```python
from build123d import *

# Parameters (mm, degrees)
SKETCH_1_R      = 1.65
EXTRUDE_1_DEPTH = 4.5


with BuildPart() as part:
    # 草图1 → 凸台-拉伸1 (new body)
    with BuildSketch(Plane.XY):
        with BuildLine():
            Line((7985.952332202, 5156.773837904), (7985.952332202, 5150.976359203))
            ThreePointArc((7985.952332202, 5150.976359203), (7986.043696587, 5150.147298626), (7986.313404682, 5149.358029069))
            Line((7986.313404682, 5149.358029069), (7993.434341187, 5134.194369164))
            ThreePointArc((7993.434341187, 5134.194369164), (8000.767739464, 5133.728654178), (7997.228995286, 5140.168600636))
            Line((7997.228995286, 5140.168600636), (7997.228995286, 5144.169137786))
            ThreePointArc((7997.228995286, 5144.169137786), (7998.107674943, 5146.290458129), (8000.228995286, 5147.169137786))
            Line((8000.228995286, 5147.169137786), (8057.335847124, 5147.169137786))
            ThreePointArc((8057.335847124, 5147.169137786), (8059.457167467, 5146.290458129), (8060.335847124, 5144.169137786))
            Line((8060.335847124, 5144.169137786), (8060.335847124, 5140.181434516))
            ThreePointArc((8060.335847124, 5140.181434516), (8056.672629109, 5133.729954227), (8064.072159737, 5134.266340868))
            Line((8064.072159737, 5134.266340868), (8071.275990148, 5149.357818804))
            ThreePointArc((8071.275990148, 5149.357818804), (8071.552278457, 5150.153987911), (8071.645915883, 5150.991515528))
            Line((8071.645915883, 5150.991515528), (8071.645915883, 5156.773837904))
            ThreePointArc((8071.645915883, 5156.773837904), (8070.767236227, 5158.895158248), (8068.645915883, 5159.773837904))
            Line((8068.645915883, 5159.773837904), (7988.952332202, 5159.773837904))
            ThreePointArc((7988.952332202, 5159.773837904), (7986.831011858, 5158.895158248), (7985.952332202, 5156.773837904))
        make_face()
        with Locations((7997.228995286, 5135.976359203)):
            Circle(SKETCH_1_R, mode=Mode.SUBTRACT)
        with Locations((8005.228995286, 5150.976359203)):
            Circle(SKETCH_1_R, mode=Mode.SUBTRACT)
        with Locations((8052.228995286, 5150.976359203)):
            Circle(SKETCH_1_R, mode=Mode.SUBTRACT)
        with Locations((8013.728995286, 5150.976359203)):
            Circle(SKETCH_1_R, mode=Mode.SUBTRACT)
        with Locations((8043.728995286, 5150.976359203)):
            Circle(SKETCH_1_R, mode=Mode.SUBTRACT)
        with Locations((8060.228995286, 5135.976359203)):
            Circle(SKETCH_1_R, mode=Mode.SUBTRACT)
        with Locations((7989.759553619, 5150.976359203)):
            Circle(SKETCH_1_R, mode=Mode.SUBTRACT)
        with Locations((8067.903645142, 5150.680599992)):
            Circle(SKETCH_1_R, mode=Mode.SUBTRACT)
        with Locations((8025.728995286, 5150.976359203)):
            Circle(SKETCH_1_R, mode=Mode.SUBTRACT)
        with Locations((8031.728995286, 5150.976359203)):
            Circle(SKETCH_1_R, mode=Mode.SUBTRACT)
        with Locations((8005.228995286, 5156.218532456)):
            Circle(SKETCH_1_R, mode=Mode.SUBTRACT)
        with Locations((8052.228995286, 5156.218532456)):
            Circle(SKETCH_1_R, mode=Mode.SUBTRACT)
        with Locations((8013.728995286, 5156.218532456)):
            Circle(SKETCH_1_R, mode=Mode.SUBTRACT)
        with Locations((8043.728995286, 5156.218532456)):
            Circle(SKETCH_1_R, mode=Mode.SUBTRACT)
        with Locations((7989.759553619, 5156.218532456)):
            Circle(SKETCH_1_R, mode=Mode.SUBTRACT)
        with Locations((8067.903645142, 5155.922773245)):
            Circle(SKETCH_1_R, mode=Mode.SUBTRACT)
        with Locations((8025.728995286, 5156.218532456)):
            Circle(SKETCH_1_R, mode=Mode.SUBTRACT)
        with Locations((8031.728995286, 5156.218532456)):
            Circle(SKETCH_1_R, mode=Mode.SUBTRACT)
    extrude(amount=EXTRUDE_1_DEPTH)


solid = part.part
```
Input: part model. Units: mm. Frame: model coordinates. A direction names the side the tool comes from. Round coordinates to 2 decimals unless told otherwise and drop trailing zeros. Loops run counter-clockwise (first coordinate to the right, second up) from the corner with the lowest first, then second, coordinate; pieces in that order, holes last. Notation, with made-up numbers: (88, 28.25) -> (105, 28.25) arc R15 ccw to (105, 43.25) -> close; hole circle Ø5 at (-8, 14.5). An arc over 180 degrees is marked (long way). Write each question's results on one line, items separated by ' | '.
1. Section D-D (x = 8023). Return loops of the section in (y, z), and give its area (3 significant figures).
Geometry results:
outline: (5147.17, 0) -> (5159.77, 0) -> (5159.77, 4.5) -> (5147.17, 4.5) -> close | area: 56.7 mm2
2. Mould query, pull axis X, two halves, no side actions, for faces 3 (the face through (7985.952, 5154, 2)), 4 (the face through (8028, 5147.169, 2)), 5 (the face through (8071.55, 5150.14, 2.22)). Classes: +X half, -X half, draft (parallel to the pull), parting line (faces both ways), or undercut.
Geometry results:
face 3: -X half | face 4: undercut | face 5: +X half
3. Section B-B (y = 5143). Return loops of the section in (x, z).
Geometry results:
outline: (7989.3, 0) -> (7997.23, 0) -> (7997.23, 4.5) -> (7989.3, 4.5) -> close; (8060.34, 0) -> (8068.24, 0) -> (8068.24, 4.5) -> (8060.34, 4.5) -> close
4. First-contact query: P1, Ø5.5, axis at x = 8031.73, y = 5156.22, coming from the +Z side; P2, Ø1, axis at y = 5146.5, z = 2.5, coming from the +X side. Flat tips, straight axial feed; report the tip coordinate or a pass-through.
Geometry results:
P1: z = 4.5 | P2: x = 8070.15
5. Ray query, line 1 (Y direction, x = 8013.5, z = 1.7); line 2 (Y direction, x = 8060, z = 4.2); line 3 (Y direction, x = 8047, z = 1.9). Return the intervals inside material, ascending. Write a range as from..to.
Geometry results:
line 1: 5147.17..5149.34, 5152.61..5154.58, 5157.85..5159.77 | line 2: 5131.78..5134.34, 5137.61..5140.18, 5145.55..5159.77 | line 3: 5147.17..5159.77
6. Section C-C (z = 3.25). State how many separate pieces and enclosed holes the cut face has, and give its area (3 significant figures).
Geometry results:
separate pieces: 1 | enclosed holes: 18 | area: 1,170 mm2
7. Section A-A (x = 8043). Return loops of the section in (y, z).
Geometry results:
outline: (5147.17, 0) -> (5149.5, 0) -> (5149.5, 4.5) -> (5147.17, 4.5) -> close; (5152.46, 0) -> (5154.74, 0) -> (5154.74, 4.5) -> (5152.46, 4.5) -> close; (5157.7, 0) -> (5159.77, 0) -> (5159.77, 4.5) -> (5157.7, 4.5) -> close
8. Set-up query: faces 1 (the face through (7989.824, 5141.882, 2.218)), 2 (the face through (7998.084, 5146.267, 2.218)). Return all of +Z, -Z, +X, -X, +Y, -Y with unobstructed straight access to the full face (end or side cutting, diameter ignored); none if empty.
Geometry results:
face 1: +Z, -Z, -X, -Y | face 2: +Z, -Z
